Could you check a few things on this model? Use its own coordinates, in mm. A direction names the side the tool comes from. Give positions to 0.01 mm unless a question says otherwise; leave off trailing zeros. Order: outer loops, then holes, each group sorted by start corner. A loop starts at its lowest first (then second) coordinate and runs counter-clockwise, first axis right, second up. Notation, with made-up numbers: (65.5, 61.5) -> (88.5, 61.5) arc R35 cw to (88.5, 100.5) -> close; hole circle Ø9 at (47, -4). An arc over 180 degrees is marked (long way). One line per item, written item: value.
```python
from build123d import *

# Parameters (mm, degrees)
F0_R     = 1
F0_R_2   = 2
F1_DEPTH = 1.5
F2_SCALE = 10


# Not quite as in the source:
# - ends of sketch curves that miss each other by under 0.0002 mm in the source are joined


with BuildPart() as f1:
    # F0 (on Top) → F1 (new body)
    with BuildSketch(Plane.XY):
        with BuildLine():
            ThreePointArc((14.156854, 15), (13.3914871353, 14.847759065), (12.7426404376, 14.4142135624))
            Line((12.7426404376, 14.4142135624), (11.414213, 13.085786))
            ThreePointArc((11.414213, 13.085786), (10.7653665381, 12.6522407997), (10, 12.5))
            Line((10, 12.5), (-10, 12.5))
            ThreePointArc((-10, 12.5), (-10.7653668647, 12.652240935), (-11.4142135624, 13.0857864376))
            Line((-11.4142135624, 13.0857864376), (-12.742641, 14.414213))
            ThreePointArc((-12.742641, 14.414213), (-13.3914871353, 14.847759065), (-14.156854, 15))
            Line((-14.156854, 15), (-20, 15))
            Line((-20, 15), (-20, -15))
            Line((-20, -15), (-14.156854, -15))
            ThreePointArc((-14.156854, -15), (-13.3914874619, -14.8477592003), (-12.7426409376, -14.4142140624))
            Line((-12.7426409376, -14.4142140624), (-11.414214, -13.085787))
            ThreePointArc((-11.414214, -13.085787), (-10.7653671914, -12.6522410703), (-10, -12.5))
            Line((-10, -12.5), (10, -12.5))
            ThreePointArc((10, -12.5), (10.7653668647, -12.652240935), (11.4142135624, -13.0857864376))
            Line((11.4142135624, -13.0857864376), (12.742641, -14.414214))
            ThreePointArc((12.742641, -14.414214), (13.3914874619, -14.8477592003), (14.156854, -15))
            Line((14.156854, -15), (20, -15))
            Line((20, -15), (20, 15))
            Line((20, 15), (14.156854, 15))
        make_face()
        with Locations((-18, -12.5)):
            Circle(F0_R, mode=Mode.SUBTRACT)
        with Locations((-18, -8.2)):
            Circle(F0_R, mode=Mode.SUBTRACT)
        with Locations((-12, -5.744006)):
            Circle(F0_R_2, mode=Mode.SUBTRACT)
        with Locations((18, -12.5)):
            Circle(F0_R, mode=Mode.SUBTRACT)
        with Locations((18, -8.2)):
            Circle(F0_R, mode=Mode.SUBTRACT)
        with Locations((12, -5.744006)):
            Circle(F0_R_2, mode=Mode.SUBTRACT)
        with Locations((-12, 0)):
            Circle(F0_R_2, mode=Mode.SUBTRACT)
        with Locations((-12, 6)):
            Circle(F0_R_2, mode=Mode.SUBTRACT)
        with Locations((-18, 8.2)):
            Circle(F0_R, mode=Mode.SUBTRACT)
        with Locations((-18, 12.5)):
            Circle(F0_R, mode=Mode.SUBTRACT)
        with BuildLine():
            ThreePointArc((-6, 5), (-5.4142135624, 6.4142135624), (-4, 7))
            Line((-4, 7), (4, 7))
            ThreePointArc((4, 7), (5.4142135624, 6.4142135624), (6, 5))
            Line((6, 5), (6, -5))
            ThreePointArc((6, -5), (5.4142135624, -6.4142135624), (4, -7))
            Line((4, -7), (-4, -7))
            ThreePointArc((-4, -7), (-5.4142135624, -6.4142135624), (-6, -5))
            Line((-6, -5), (-6, 5))
        make_face(mode=Mode.SUBTRACT)
        with Locations((12, 0)):
            Circle(F0_R_2, mode=Mode.SUBTRACT)
        with Locations((12, 6)):
            Circle(F0_R_2, mode=Mode.SUBTRACT)
        with Locations((18, 8.2)):
            Circle(F0_R, mode=Mode.SUBTRACT)
        with Locations((18, 12.5)):
            Circle(F0_R, mode=Mode.SUBTRACT)
    extrude(amount=F1_DEPTH)


with BuildPart() as f1_1:
    # F2: moved
    add(f1.part.scale(F2_SCALE).moved(Location((180, 135, -13.5))))


solid = f1_1.part
```
1) Suppose I cut it at D-D, the plane x = 60. Write out the boundary of the cut face in (y, z), then the cut area to 3 significant figures.
Answer below:
outline: (-1.72, -13.5) -> (57.56, -13.5) -> (57.56, 1.5) -> (-1.72, 1.5) -> close; (97.56, -13.5) -> (115, -13.5) -> (115, 1.5) -> (97.56, 1.5) -> close; (155, -13.5) -> (175, -13.5) -> (175, 1.5) -> (155, 1.5) -> close; (215, -13.5) -> (271.72, -13.5) -> (271.72, 1.5) -> (215, 1.5) -> close
area: 2,300 mm2
2) Suppose I cut it at A-A, the plane x = 0. Write out the boundary of the cut face in (y, z).
Answer below:
outline: (-15, -13.5) -> (0, -13.5) -> (0, 1.5) -> (-15, 1.5) -> close; (20, -13.5) -> (43, -13.5) -> (43, 1.5) -> (20, 1.5) -> close; (63, -13.5) -> (207, -13.5) -> (207, 1.5) -> (63, 1.5) -> close; (227, -13.5) -> (250, -13.5) -> (250, 1.5) -> (227, 1.5) -> close; (270, -13.5) -> (285, -13.5) -> (285, 1.5) -> (270, 1.5) -> close
3) If I drill on line 1 along X through (y, z) = (135.5, -6.5); line 2 along Y through (x, z) = (60, -9.25); line 3 along X through (y, z) = (168, -8.75), over which ranges is the centre line in solid material (lowest first)?
Answer below:
line 1: x = -20 to 40.01, 79.99 to 120, 240 to 280.01, 319.99 to 380
line 2: y = -1.72 to 57.56, 97.56 to 115, 155 to 175, 215 to 271.72
line 3: x = -20 to 120, 240 to 380
4) Suppose I cut it at B-B, the plane y = 135. Write out the boundary of the cut face in (x, z), then the cut area to 3 significant figures.
Answer below:
outline: (-20, -13.5) -> (40, -13.5) -> (40, 1.5) -> (-20, 1.5) -> close; (80, -13.5) -> (120, -13.5) -> (120, 1.5) -> (80, 1.5) -> close; (240, -13.5) -> (280, -13.5) -> (280, 1.5) -> (240, 1.5) -> close; (320, -13.5) -> (380, -13.5) -> (380, 1.5) -> (320, 1.5) -> close
area: 3,000 mm2
5) For P1, Ø1.5, axis at x = 159.5, z = -1, coming from the -Y side; P2, Ø7.5, axis at x = 132, z = -4, coming from the +Y side; P3, Ø8, axis at x = 71, z = -9, coming from the +Y side, each with a flat end and sliding along its axis, tell me the tip position at first contact or that it passes through.
Answer below:
P1: stops at y = 10
P2: stops at y = 260
P3: stops at y = 264.8
6) For faces 1 (the flat face through (179, 205, -6)), 2 (the flat face through (351, 285, -6)), 3 (the cylindrical face through (45.98, -13.52, -6.1)), 4 (the cylindrical face through (46.187, 283.435, -6.105)), which set-ups out of +Z, -Z, +X, -X, +Y, -Y let a thin tool reach every point of the face, with its end or its side?
Answer below:
face 1: +Z, -Z
face 2: +Z, -Z, +X, -X, +Y
face 3: +Z, -Z, -Y
face 4: +Z, -Z, +Y
7) Suppose I cut it at C-C, the plane y = 53. Write out the boundary of the cut face in (x, z), then the cut area to 3 significant figures.
Answer below:
outline: (-20, -13.5) -> (-10, -13.5) -> (-10, 1.5) -> (-20, 1.5) -> close; (10, -13.5) -> (350, -13.5) -> (350, 1.5) -> (10, 1.5) -> close; (370, -13.5) -> (380, -13.5) -> (380, 1.5) -> (370, 1.5) -> close
area: 5,400 mm2
8) We'd pull the mould along X, two halves only. Please class faces 5 (the flat face through (380, 133, -6)), 6 (the flat face through (133, 204, -13.5)), 7 (the flat face through (120, 134, -6)): +X half, -X half, draft (parallel to the pull), parting line (faces both ways), or undercut.
Answer below:
face 5: +X half
face 6: draft
face 7: undercut
